Geometry: final body of the model. Coordinates: model frame, mm. Face numbers are marked on the shaded views. A direction names the side the tool comes from. Give positions to 0.01 mm unless a question says otherwise; leave off trailing zeros. Order: outer loops, then holes, each group sorted by start corner. A loop starts at its lowest first (then second) coordinate and runs counter-clockwise, first axis right, second up. Notation, with made-up numbers: (-38, 86) - (-29, 86) arc R21 ccw to (-29, 107) - close; hole circle Ø8 at (65.5, -28). An arc over 180 degrees is marked (long way). Put each result on its own line as item: value. Start each with the question number.
1. Section D-D on x = -5.5. Return the cut outline in (y, z) (3 decimals), plus the area to 3 significant figures.
2. Set-up query: the marked faces 1, 2 and 3. Return all of +Z, -Z, +X, -X, +Y, -Y with unobstructed straight access to the full face (end or side cutting, diameter ignored); none if empty.
3. Section A-A on z = 0. Return the cut outline in (x, y) (3 decimals), plus the area to 3 significant figures.
4. Ray query, line 1 along X through (y, z) = (-5.5, 3.5); line 2 along X through (y, z) = (-7.5, -4.5); line 3 along X through (y, z) = (-4, -1). Return the intervals inside material, ascending. Write a range as from..to.
5. First-contact query: P1, Ø1.5, axis at x = -7, z = 7, coming from the +Y side; P2, Ø2, axis at y = 5.5, z = -2.5, coming from the -X side; P3, Ø1.5, axis at x = -22, y = 2, coming from the +Z side. Flat tips, straight axial feed; report the tip coordinate or a pass-through.
6. Mould query, pull axis X, two halves, no side actions, for the marked faces 4, 5 and 6. Classes: pulls with the +X half, pulls with the -X half, needs draft (parallel to the pull), parting line crosses it, or undercut.
7. Section C-C on x = -26. Return the cut outline in (y, z) (3 decimals), plus the area to 3 significant figures.
from build123d import *


with BuildPart() as f1:
    # F0 (on Front) → F1 (revolve)
    with BuildSketch(Plane.XZ):
        with BuildLine():
            Line((-31.406309, 0), (-3.212309, 0))
            Line((-3.212309, 0), (-3.212309, 9.525))
            Line((-3.212309, 9.525), (-8.800309, 9.525))
            Line((-8.800309, 9.525), (-13.236284, 5.089026))
            ThreePointArc((-13.236284, 5.089026), (-14.134309, 4.717051), (-15.032335, 5.089026))
            Line((-15.032335, 5.089026), (-19.468309, 9.525))
            Line((-19.468309, 9.525), (-25.056309, 9.525))
            Line((-25.056309, 9.525), (-25.056309, 3.175))
            Line((-25.056309, 3.175), (-31.406309, 3.175))
            Line((-31.406309, 3.175), (-31.406309, 0))
        make_face()
    revolve(axis=Axis((-44.154793, 0, 0), (1, 0, 0)))


solid = f1.part
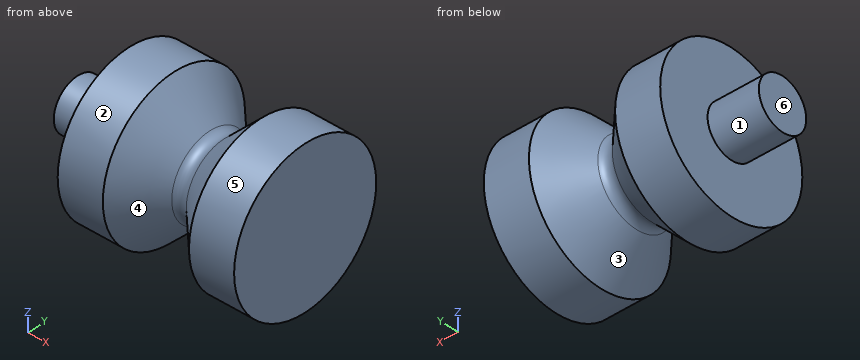
Resolved:
1. outline: circle Ø19.05 at (0, 0)
1. area: 285 mm^2
2. face 1: -X
2. face 2: +X, -X
2. face 3: none
3. outline: (-31.406, -3.175) - (-25.056, -3.175) - (-25.056, -9.525) - (-19.468, -9.525) - (-15.032, -5.089) arc R1.27 cw to (-13.236, -5.089) - (-8.8, -9.525) - (-3.212, -9.525) - (-3.212, 9.525) - (-8.8, 9.525) - (-13.236, 5.089) arc R1.27 cw to (-15.032, 5.089) - (-19.468, 9.525) - (-25.056, 9.525) - (-25.056, 3.175) - (-31.406, 3.175) - close
3. area: 400 mm^2
4. line 1: -25.06..-16.46, -11.81..-3.21
4. line 2: -25.06..-18.69, -9.58..-3.21
4. line 3: -25.06..-3.21
5. P1: y = 7.19
5. P2: x = -25.06
5. P3: z = 9.44
6. face 4: undercut
6. face 5: needs draft
6. face 6: pulls with the -X half
7. outline: circle Ø6.35 at (0, 0)
7. area: 31.7 mm^2
